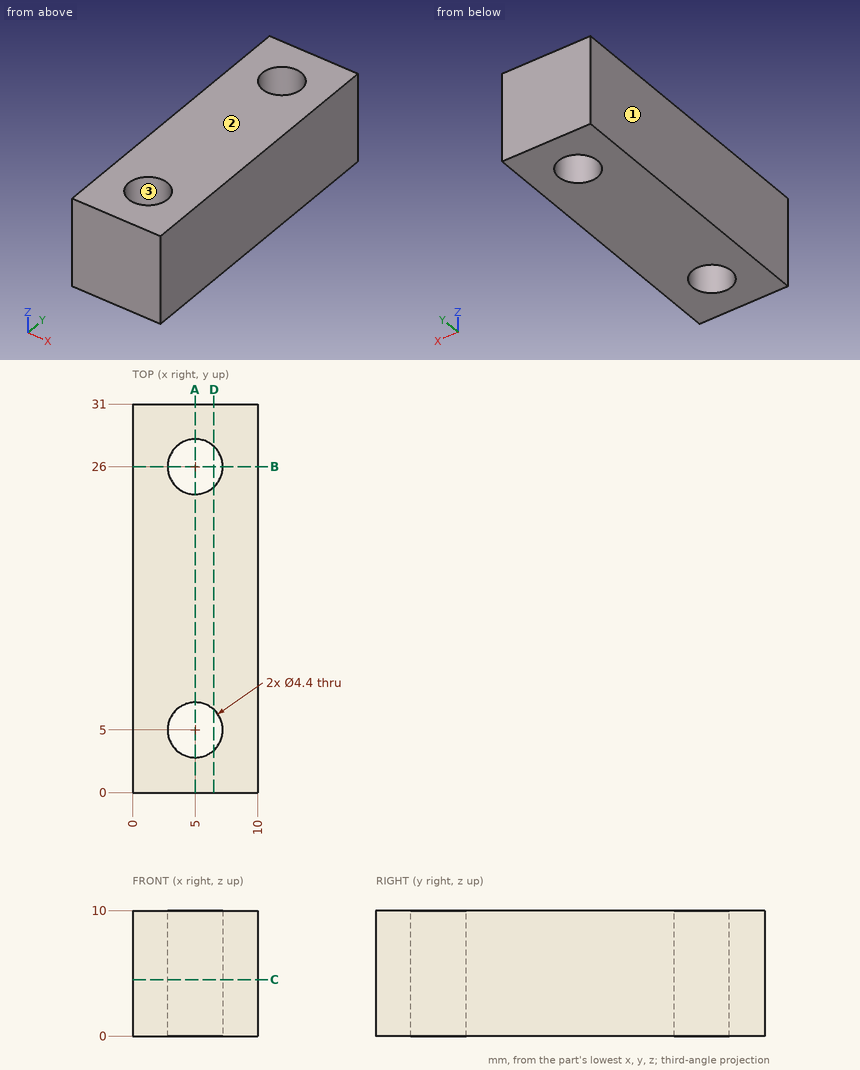
Verification items for this drawing (mm, ordinates from the low corner). Round coordinates to 2 decimals unless told otherwise and drop trailing zeros. Order: outer loops, then holes, each group sorted by start corner. A loop starts at its lowest first (then second) coordinate and runs counter-clockwise, first axis right, second up.
1) Material ranges on line 1 (Y direction, x = 5, z = 5); line 2 (Y direction, x = 6.5, z = 1.75); line 3 (X direction, y = 4, z = 6.75), recorded low to high.
Geometry says:
line 1: y = 0 to 2.8, 7.2 to 23.8, 28.2 to 31
line 2: y = 0 to 3.39, 6.61 to 24.39, 27.61 to 31
line 3: x = 0 to 3.04, 6.96 to 10
2) Cross-section at C-C, the plane z = 4.5. Record the cut outline in (x, y), plus the area to 3 significant figures.
Geometry says:
outline: (0, 0) - (10, 0) - (10, 31) - (0, 31) - close; hole circle Ø4.4 at (5, 5); hole circle Ø4.4 at (5, 26)
area: 280 mm2
3) Cross-section at D-D, the plane x = 6.5. Record the cut outline in (y, z), plus the area to 3 significant figures.
Geometry says:
outline: (0, 0) - (3.39, 0) - (3.39, 10) - (0, 10) - close; (6.61, 0) - (24.39, 0) - (24.39, 10) - (6.61, 10) - close; (27.61, 0) - (31, 0) - (31, 10) - (27.61, 10) - close
area: 246 mm2
4) Cross-section at B-B, the plane y = 26. Record the cut outline in (x, z), plus the area to 3 significant figures.
Geometry says:
outline: (0, 0) - (2.8, 0) - (2.8, 10) - (0, 10) - close; (7.2, 0) - (10, 0) - (10, 10) - (7.2, 10) - close
area: 56.0 mm2
5) Cross-section at A-A, the plane x = 5. Record the cut outline in (y, z).
Geometry says:
outline: (0, 0) - (2.8, 0) - (2.8, 10) - (0, 10) - close; (7.2, 0) - (23.8, 0) - (23.8, 10) - (7.2, 10) - close; (28.2, 0) - (31, 0) - (31, 10) - (28.2, 10) - close
6) Draft check along X on the marked faces 1, 2 and 3. Enter one of: +X half, -X half, draft (parallel to the pull), parting line (faces both ways), or undercut.
Geometry says:
face 1: -X half
face 2: draft
face 3: undercut
7) Depth check by flat-ended pin: pin 1 (6 mm diameter, centred on x = 6.5, y = 21.5, fed in from -Z). Enter the tip coordinate at first touch or a pass-through.
Geometry says:
pin 1: stops at z = 0
